Autodesk Inventor part; units mm, degrees
ref_plane "YZ Plane" through (0, 0, 0) normal (1, 0, 0) x (0, 1, 0)
ref_plane "XZ Plane" through (0, 0, 0) normal (0, 1, 0) x (-1, 0, 0)
ref_plane "XY Plane" through (0, 0, 0) normal (0, 0, 1) x (1, 0, 0)
sketch "Sketch1" plane through (0, 0, 0) normal (0, 0, 1) x (1, 0, 0)
  line L0 (0, 8.6995) -> (0, 0)
  line L1 (0, 0) -> (2.8194, 0)
  line L2 (2.8194, 0) -> (2.7559, 1.1684)
  line L3 (2.7559, 1.1684) -> (2.4384, 1.1684)
  line L4 (2.4384, 1.1684) -> (2.4384, 6.2611)
  arc A0 (2.4384, 6.2611) -> (0, 8.6995) centre (0, 6.2611) ccw
  dimension "d0" = 2.4384
  dimension "d1" = 2.8194
  dimension "d2" = 2.7559
  dimension "d3" = 1.1684
  dimension "d4" = 8.6995
revolve "Revolution1" add sketch "Sketch1" angle 360 about axis through (0, 8.6995, 0) along (0, -1, 0)
sketch "Sketch2" plane through (0, 0, 0) normal (0, -1, 0) x (1, 0, 0)
  line L0 (0.235, 2.1273) -> (-0.2349, 2.1273)
  line L1 (-0.2349, 2.1273) -> (-0.2349, 1.4034)
  line L2 (-0.2349, 1.4034) -> (0.235, 1.4034)
  line L3 (0.235, 1.4034) -> (0.235, 2.1273)
  line L4 (0.235, 2.1273) -> (-0.2349, 1.4034) construction
  line L5 (-0.2349, 2.1273) -> (0.235, 1.4034) construction
  line L6 (0.235, 0.9504) -> (-0.2349, 0.9504)
  line L7 (-0.2349, 0.9504) -> (-0.2349, 0.2265)
  line L8 (-0.2349, 0.2265) -> (0.235, 0.2265)
  line L9 (0.235, 0.2265) -> (0.235, 0.9504)
  line L10 (0.235, 0.9504) -> (-0.2349, 0.2265) construction
  line L11 (-0.2349, 0.9504) -> (0.235, 0.2265) construction
  line L12 (0.235, -0.2265) -> (-0.2349, -0.2265)
  line L13 (-0.2349, -0.2265) -> (-0.2349, -0.9504)
  line L14 (-0.2349, -0.9504) -> (0.235, -0.9504)
  line L15 (0.235, -0.9504) -> (0.235, -0.2265)
  line L16 (0.235, -0.2265) -> (-0.2349, -0.9504) construction
  line L17 (-0.2349, -0.2265) -> (0.235, -0.9504) construction
  line L18 (0.2349, -1.4033) -> (-0.2349, -1.4033)
  line L19 (-0.2349, -1.4033) -> (-0.2349, -2.1273)
  line L20 (-0.2349, -2.1273) -> (0.2349, -2.1273)
  line L21 (0.2349, -2.1273) -> (0.2349, -1.4033)
  line L22 (0.2349, -1.4033) -> (-0.2349, -2.1273) construction
  line L23 (-0.2349, -1.4033) -> (0.2349, -2.1273) construction
  circle A0 centre (0, 0) radius 2.7559 construction
  line L24 (2.7559, 0) -> (-2.7559, 0) construction
  point P0 (0, 0)
  point P1 (0, 1.7653)
  point P2 (0, 0.5884)
  point P3 (0, -0.5884)
  point P4 (0, -1.7653)
  point P5 (0, -1.7653)
  point P6 (0, -0.9504)
  point P7 (0, -0.5884)
  point P8 (0, 0.5884)
  point P9 (0, 0.2265)
  point P10 (0, 1.7653)
  point P11 (0, -0.5884)
  dimension "d6" = 0.4699
  dimension "d7" = 0.7239
  dimension "d8" = 4.2545
  dimension "d9" = 0.453
  dimension "d10" = 0.453
extrude "Extrusion1" add sketch "Sketch2" along normal blind 24.7396
sketch "Sketch3" plane through (0, -24.7396, 0) normal (0, -1, 0) x (1, 0, 0)
  line L0 (0.235, 2.1273) -> (-0.2349, 2.1273)
  line L1 (-0.2349, 2.1273) -> (-0.2349, 1.4034)
  line L2 (-0.2349, 1.4034) -> (0.235, 1.4034)
  line L3 (0.235, 1.4034) -> (0.235, 2.1273)
  line L4 (0.235, -0.2265) -> (-0.2349, -0.2265)
  line L5 (-0.2349, -0.2265) -> (-0.2349, -0.9504)
  line L6 (-0.2349, -0.9504) -> (0.235, -0.9504)
  line L7 (0.235, -0.9504) -> (0.235, -0.2265)
  point P0 (0, 0)
extrude "Extrusion2" add sketch "Sketch3" along normal blind 1.2065
sketch "Sketch4" plane through (0, -24.7396, 0) normal (0, -1, 0) x (1, 0, 0)
  line L0 (0.235, 0.9504) -> (-0.2349, 0.9504)
  line L1 (-0.2349, 0.9504) -> (-0.2349, 0.2265)
  line L2 (-0.2349, 0.2265) -> (0.235, 0.2265)
  line L3 (0.235, 0.2265) -> (0.235, 0.9504)
  point P0 (0, 0)
extrude "Extrusion3" add sketch "Sketch4" along normal blind 2.0193
equation "\"d9\" = d10"
properties part number "Full LED"
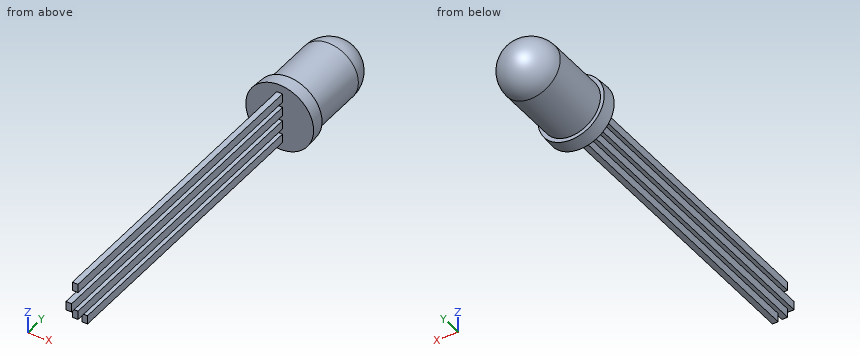
Model file for the job. Use its own axes, mm. Give positions to 0.01 mm unless a question says otherwise; leave off trailing zeros. Loops run counter-clockwise (first coordinate to the right, second up) from the corner with the lowest first, then second, coordinate; pieces in that order, holes last. Notation, with made-up numbers: (23, 30.25) -> (37, 30.25) arc R20 cw to (37, 40.25) -> close; hole circle Ø11 at (6, -30.5). An arc over 180 degrees is marked (long way). Use CSV: the item, a comma, the result in double quotes. Start each with the question number.
1) Flat gauge pins, fed straight in: pin 1 Ø3 at (x, y) = (1.5, 4.5) entering from +Z; pin 2 Ø0.5 at (x, y) = (0, -6.5) entering from -Z; pin 3 Ø3 at (x, y) = (-2, -7.5) entering from +Z; pin 4 Ø0.6 at (y, z) = (-12, -2) entering from +X. Where does each tip first touch, or does it go through?
2) Wall check: line 1 (Z direction, x = 0, y = -17.5); line 2 (X direction, y = -11, z = -0.4) (3 decimals); line 3 (Y direction, x = 0.25, z = -2.5). Give the ranges that are in metal, low to high.
3) Slice it at B-B on y = 4. Give the cut face in (x, z), plus the area to 3 significant figures.
4) Slice it at A-A on y = -0.5. Give the cut face in (x, z) (1 decimal).
Computed values:
1,pin 1,"stops at z = 2.44"
1,pin 2,"stops at z = -2.13"
1,pin 3,"passes through"
1,pin 4,"stops at x = 0.23"
2,line 1,"z = -2.13 to -1.4, -0.95 to -0.23, 0.23 to 0.95, 1.4 to 2.13"
2,line 2,"x = -0.235 to 0.235"
2,line 3,"y = 0 to 1.17"
3,outline,"circle Ø4.88 at (0, 0)"
3,area,"18.7 mm^2"
4,outline,"(-0.2, -2.1) -> (0.2, -2.1) -> (0.2, -1.4) -> (-0.2, -1.4) -> close; (-0.2, -1) -> (0.2, -1) -> (0.2, -0.2) -> (-0.2, -0.2) -> close; (-0.2, 0.2) -> (0.2, 0.2) -> (0.2, 1) -> (-0.2, 1) -> close; (-0.2, 1.4) -> (0.2, 1.4) -> (0.2, 2.1) -> (-0.2, 2.1) -> close"
